```python
from build123d import *


with BuildPart() as part:
    # Sketch1 → Revolve1 (revolve)
    with BuildSketch(Plane.XY):
        with BuildLine():
            Line((0, 45), (4, 45))
            Line((4, 45), (4, 33))
            ThreePointArc((4, 33), (5.171572875, 30.171572875), (8, 29))
            Line((8, 29), (12, 29))
            Line((12, 29), (12, 25))
            Line((12, 25), (8, 25))
            ThreePointArc((8, 25), (2.343145751, 27.343145751), (0, 33))
            Line((0, 33), (0, 45))
        make_face()
    revolve(axis=Axis((0, 0, 0), (1, 0, 0)))


solid = part.part
```
Could you check a few things on this model? Use its own coordinates, in mm. A direction names the side the tool comes from. Coordinates: 2 decimals unless noted, no trailing zeros. Write each loop counter-clockwise with the first axis right and the second up, starting at its lowest first coordinate (ties: lowest second). Pieces come first, ordered by that corner, then holes. Notation, with made-up numbers: (52.5, -12) -> (65.5, -12) arc R21 cw to (65.5, 11) -> close; hole circle Ø11 at (54.5, 61.25). An arc over 180 degrees is marked (long way). One line per question, with ' | ' between items. Start each with the question number.
1. Will these pins go through, and if not, where does the flat tip stop? P1, Ø3, axis at x = 2, z = 27, coming from the +Y side; P2, Ø3, axis at x = 7, y = -17, coming from the +Z side; P3, Ø6, axis at x = 6, z = -15, coming from the +Y side; P4, Ø1, axis at x = 6, z = 35.5, coming from the -Y side.
2. Thinking about a two-plate mould opening in Z: for faces 1 (the face through (12, 13, 22)), 2 (the face through (2.028, 20.765, -39.923)), 3 (the face through (9.972, 23.846, 7.509)), which applies, pulls with the +Z half, pulls with the -Z half, needs draft (parallel to the pull), parting line crosses it, or undercut?
3. If we section it at A-A (z = 0): Please give me the cut outline in (x, y), and give its area (3 significant figures).
4. If we section it at C-C (x = 1.25): Please give me the cut outline in (y, z).
5. For faces 4 (the face through (0, 24, 24)), 5 (the face through (10.03, 13.38, -25.73)), which set-ups out of +Z, -Z, +X, -X, +Y, -Y let a thin tool reach every point of the face, with its end or its side?
6. If we section it at D-D (y = 35): Please give me the cut outline in (x, z).
7. Please list where these lines run through material, in increasing order: line 1 along Z through (x, y) = (9.95, 0); line 2 along X through (y, z) = (-18.5, -33); line 3 along Y through (x, z) = (1, 2).
Return value:
1) P1: stops at y = 37.08 | P2: stops at z = 24.91 | P3: stops at y = 43.15 | P4: passes through
2) face 1: needs draft | face 2: parting line crosses it | face 3: undercut
3) outline: (0, -45) -> (4, -45) -> (4, -33) arc R4 cw to (8, -29) -> (12, -29) -> (12, -25) -> (8, -25) arc R8 ccw to (0, -33) -> close; (0, 33) arc R8 ccw to (8, 25) -> (12, 25) -> (12, 29) -> (8, 29) arc R4 cw to (4, 33) -> (4, 45) -> (0, 45) -> close | area: 203 mm²
4) outline: circle Ø90 at (0, 0); hole circle Ø57.41 at (0, 0)
5) face 4: +Z, -Z, -X, +Y, -Y | face 5: +X
6) outline: (0, -28.28) -> (4, -28.28) -> (4, 28.28) -> (0, 28.28) -> close
7) line 1: z = -29 to -25, 25 to 29 | line 2: x = 0 to 4 | line 3: y = -44.96 to -29.06, 29.06 to 44.96
